The listing builds one solid part. Answer for the finished solid, in the listing's coordinates (mm). Round coordinates to 2 decimals unless told otherwise and drop trailing zeros. Write each loop counter-clockwise with the first axis right and the second up, starting at its lowest first coordinate (ties: lowest second). Pieces come first, ordered by that corner, then holes. Notation, with made-up numbers: M -21.5,41 L 13.5,41 A23 cw 13.5,54 Z; hole C 23,-25 d2. An arc over 180 degrees is marked long. Write each question's results on one line, items separated by ' | '.
from build123d import *

# Parameters (mm, degrees)
AUFSATZ_LINEAR_AUSTRAGEN1_DEPTH = 4.76
SKIZZE2_R                       = 2.575
SCHNITT_LINEAR_AUSTRAGEN2_DEPTH = 4.76


with BuildPart() as part:
    # Skizze1 → Aufsatz-Linear austragen1 (new body)
    with BuildSketch(Plane(origin=(0, 0, 0), x_dir=(1, 0, 0), z_dir=(0, 1, 0))):
        with BuildLine():
            Line((1.637816376, 6.35), (10.594588216, 1.400399316))
            ThreePointArc((10.594588216, 1.400399316), (11.420713706, 0), (10.594588216, -1.400399316))
            Line((10.594588216, -1.400399316), (1.637816376, -6.35))
            Line((1.637816376, -6.35), (-1.637816376, -6.35))
            Line((-1.637816376, -6.35), (-10.594588216, -1.400399316))
            ThreePointArc((-10.594588216, -1.400399316), (-11.420713706, 0), (-10.594588216, 1.400399316))
            Line((-10.594588216, 1.400399316), (-1.637816376, 6.35))
            Line((-1.637816376, 6.35), (1.637816376, 6.35))
        make_face()
    extrude(amount=AUFSATZ_LINEAR_AUSTRAGEN1_DEPTH)

    # Skizze2 → Schnitt-Linear austragen2 (cut)
    with BuildSketch(Plane(origin=(0, 0, 0), x_dir=(-1, 0, 0), z_dir=(0, -1, 0))):
        with Locations(Location((0, 0, 0), (0, 0, 90))):  # turned: the seam where the file's is
            Circle(SKIZZE2_R)
    extrude(amount=-SCHNITT_LINEAR_AUSTRAGEN2_DEPTH, mode=Mode.SUBTRACT)


solid = part.part
1) Each of these flat-tipped pins is pushed along its axis until it touches: pin 1 (4 mm diameter, centred on x = 0, z = 0, fed in from -Y); pin 2 (1.5 mm diameter, centred on y = 3.5, z = -4.5, fed in from +X). Where does it stop, or does it pass through?
Return value:
pin 1: through | pin 2: x = 6.34
2) Find the intervals of material crossed by line 1 (Z direction, x = -0.75, y = 3.5); line 2 (X direction, y = 0.3, z = -0.5); line 3 (Z direction, x = 6.5, y = 3.2), in increasing order.
Return value:
line 1: -6.35 to -2.46, 2.46 to 6.35 | line 2: -11.34 to -2.53, 2.53 to 11.34 | line 3: -3.66 to 3.66
3) The mould has two halves that part along Z. Classify faces 1 (the face through (-11.42, 2.35, 0.02)), 2 (the face through (3, 0, 0)), 3 (the face through (-2.514, 2.347, 0.558)): +Z half, -Z half, draft (parallel to the pull), parting line (faces both ways), or undercut.
Return value:
face 1: parting line | face 2: draft | face 3: undercut
4) Section A-A (x = 0) is taken. Determine the outline of the cut face in (y, z) (3 decimals).
Return value:
outline: M 0,-6.35 L 4.76,-6.35 L 4.76,-2.575 L 0,-2.575 Z; M 0,2.575 L 4.76,2.575 L 4.76,6.35 L 0,6.35 Z
5) Section C-C (y = 3.15) is taken. Determine the outline of the cut face in (x, z) (3 decimals).
Return value:
outline: M -10.595,-1.4 L -1.638,-6.35 L 1.638,-6.35 L 10.595,-1.4 A1.6 ccw 10.595,1.4 L 1.638,6.35 L -1.638,6.35 L -10.595,1.4 A1.6 ccw Z; hole C 0,0 d5.15
6) Section B-B (z = 0) is taken. Determine the outline of the cut face in (x, y) (3 decimals).
Return value:
outline: M -11.421,0 L -2.575,0 L -2.575,4.76 L -11.421,4.76 Z; M 2.575,0 L 11.421,0 L 11.421,4.76 L 2.575,4.76 Z
7) Section D-D (x = 10) is taken. Determine the outline of the cut face in (y, z), then the cut area to 3 significant figures.
Return value:
outline: M 0,-1.73 L 4.76,-1.73 L 4.76,1.73 L 0,1.73 Z | area: 16.5 mm²
